The listing builds one solid part. Answer for the finished solid, in the listing's coordinates (mm). A direction names the side the tool comes from. Give positions to 0.01 mm unless a question says otherwise; leave off trailing zeros. Write each loop counter-clockwise with the first axis right and the second up, starting at its lowest first coordinate (ties: lowest second). Pieces come first, ordered by that corner, then holes. Notation, with made-up numbers: (73, 0) -> (108, 0) arc R22 ccw to (108, 24) -> close; hole circle Ø3 at (40.25, 8). An arc over 180 degrees is marked (long way). Write each question's results on one line, items separated by ' | '. Start each with the question number.
from build123d import *

# Parameters (mm, degrees)
F0_W     = 61.3819211721
F0_H     = 36.4417210221
F1_DEPTH = 38.1
F2_T     = -2.54
F3_DEPTH = 7.62
F4_W     = 2.54
F4_H     = 36.4417210221
F5_DEPTH = 50.8
F6_W     = 4.7011679959
F6_H     = 4.0546688199
F6_H_2   = 4.4637494721
F6_W_2   = 4.3158759363
F7_DEPTH = 2.54


with BuildPart() as f1:
    # F0 (on Front) → F1 (new body)
    with BuildSketch(Plane.XZ):
        with Locations((30.6909605861, 18.2208605111)):
            Rectangle(F0_W, F0_H)
    extrude(amount=F1_DEPTH)

    # F2
    f2_openings = [f1.faces().sort_by_distance(p)[0] for p in [
        (30.690961, -38.1, 18.220861),
    ]]
    offset(amount=F2_T, openings=f2_openings)

    # F3 (add): a face of the model
    f3_faces = [f1.faces().sort_by_distance(p)[0] for p in [
        (61.3819211721, -19.05, 18.2208605111),
    ]]
    extrude(f3_faces, amount=F3_DEPTH)

    # F4 (on face) → F5 (join)
    with BuildSketch(Plane.XZ.offset(38.1)):
        with Locations((1.27, 18.2208605111)):
            Rectangle(F4_W, F4_H)
    extrude(amount=F5_DEPTH)

    # F6 (on face) → F7 (join)
    with BuildSketch(Plane(origin=(0, 0, 0), x_dir=(1, 0, 0), z_dir=(0, 0, -1))):
        Polygon((4.3158759363, 38.1), (2.54, 38.1), (0, 38.1), (0, 34.0453311801), (4.3158759363, 34.0453311801), align=None)
        with Locations((66.6513371742, 36.07266559)):
            Rectangle(F6_W, F6_H)
        with Locations((66.6513371742, 2.231874736)):
            Rectangle(F6_W, F6_H_2)
        with Locations((2.1579379681, 2.231874736)):
            Rectangle(F6_W_2, F6_H_2)
    extrude(amount=F7_DEPTH)


solid = f1.part
1. Section A-A (y = -24.5) is taken. Write down the section's boundary in (x, z).
2. Section D-D (y = -71) is taken. Write down the section's boundary in (x, z).
3. Section C-C (z = 17) is taken. Write down the section's boundary in (x, y).
4. Section B-B (x = 29.5) is taken. Write down the section's boundary in (y, z).
5. Consider probe 1 along X at (y, z) = (-9.5, 17); probe 2 along Z at (x, y) = (36.5, -19); probe 3 along Y at (x, z) = (57, 31.5). Determine where each line is inside the solid, lowest interval first. Write a range as [from, to].
6. The mould has two halves that part along Y. Classify faces 1 (the flat face through (1, -88.9, 18)), 2 (the flat face through (67, -4.464, -1)), 3 (the flat face through (30, -20, 33.902)), 4 (the flat face through (2, -4.464, -1)): pulls with the +Y half, pulls with the -Y half, needs draft (parallel to the pull), parting line crosses it, or undercut.
7. A tool of negligible diameter and unlimited length cuts with its end or side. For faces 5 (the flat face through (2.54, -45, 18)), 6 (the flat face through (4.316, -36, -1)), 7 (the flat face through (2, -34.045, -1)), 8 (the flat face through (2, -2, -2.54)), 9 (the flat face through (69.002, -19, 17)), from which of +Z, -Z, +X, -X, +Y, -Y can it reach the whole face along a straight path? Write none if from no direction.
8. Each of these flat-tipped pins is pushed along its axis until it touches: pin 1 Ø1 at (x, z) = (33.5, 29.5) entering from -Y; pin 2 Ø1.3 at (x, z) = (67.5, -0.5) entering from -Y; pin 3 Ø5 at (x, y) = (36, -20.5) entering from -Z. Where does it stop, or does it pass through?
Results:
1) outline: (0, 0) -> (69, 0) -> (69, 36.44) -> (0, 36.44) -> close; hole (2.54, 2.54) -> (58.84, 2.54) -> (58.84, 33.9) -> (2.54, 33.9) -> close
2) outline: (0, 0) -> (2.54, 0) -> (2.54, 36.44) -> (0, 36.44) -> close
3) outline: (0, -88.9) -> (2.54, -88.9) -> (2.54, -2.54) -> (58.84, -2.54) -> (58.84, -38.1) -> (69, -38.1) -> (69, 0) -> (0, 0) -> close
4) outline: (-38.1, 0) -> (0, 0) -> (0, 36.44) -> (-38.1, 36.44) -> (-38.1, 33.9) -> (-2.54, 33.9) -> (-2.54, 2.54) -> (-38.1, 2.54) -> close
5) probe 1: x = [0, 2.54], [58.84, 69] | probe 2: z = [0, 2.54], [33.9, 36.44] | probe 3: y = [-2.54, 0]
6) face 1: pulls with the -Y half | face 2: undercut | face 3: needs draft | face 4: undercut
7) face 5: -Y | face 6: -Z, +Y, -Y | face 7: -Z, +X, -X | face 8: -Z, +X, -X, +Y, -Y | face 9: +Z, -Z, +X, +Y, -Y
8) pin 1: stops at y = -2.54 | pin 2: stops at y = -38.1 | pin 3: stops at z = 0
